For this review, take the finished solid that the model builds, in its own axes (mm). Face numbers are marked on the shaded views. A direction names the side the tool comes from. Round coordinates to 2 decimals unless told otherwise and drop trailing zeros. Loops run counter-clockwise (first coordinate to the right, second up) from the corner with the lowest first, then second, coordinate; pieces in that order, holes last.
```python
from build123d import *
from build123d.topology import SkipClean

# Parameters (mm, degrees)
ESQUISSE1_R             = 17.5
ESQUISSE1_R_2           = 7.5
ESQUISSE1_R_3           = 10
ESQUISSE1_R_4           = 3
BOSS_EXTRU_1_DEPTH      = 11
BOSS_EXTRU_2_DEPTH      = 15.5
BOSS_EXTRU_2_DEPTH_BACK = 4.5
ESQUISSE1_3_R           = 17.5
ESQUISSE1_3_R_2         = 7.5
ESQUISSE1_3_R_3         = 10
ESQUISSE1_3_R_4         = 3


with BuildPart() as part:
    # Esquisse1 → Boss.-Extru.1 (new body)
    # profile 1 of 3: a face of its own
    with BuildSketch(Plane.XY):
        with BuildLine():
            Line((46.99759236, 11.06690166), (2.435529267, 17.329691203))
            ThreePointArc((2.435529267, 17.329691203), (13.207417654, 11.481033007), (17.5, 0))
            ThreePointArc((17.5, 0), (14.881876713, -9.207591731), (7.810886229, -15.660142283))
            Line((7.810886229, -15.660142283), (43.63238408, -12.07959879))
            Line((43.63238408, -12.07959879), (50.273258771, -18.558335793))
            ThreePointArc((50.273258771, -18.558335793), (54.140410924, -6.679083669), (66.578967785, -7.842612783))
            Line((66.578967785, -7.842612783), (46.99759236, 11.06690166))
        make_face()
    # profile 2 of 3: a face of its own
    with BuildSketch(Plane.XY):
        Circle(ESQUISSE1_R)
        Circle(ESQUISSE1_R_2, mode=Mode.SUBTRACT)
    # profile 3 of 3: a face of its own
    with BuildSketch(Plane.XY):
        with Locations((59.63238408, -15.036010787)):
            Circle(ESQUISSE1_R_3)
        with Locations((59.63238408, -15.036010787)):
            Circle(ESQUISSE1_R_4, mode=Mode.SUBTRACT)
    extrude(amount=BOSS_EXTRU_1_DEPTH)

    # Esquisse1_3 → Boss.-Extru.2 (add, two sides: drawn at the far end of the back side and taken through both)
    # profile 1 of 2: a face of its own
    with SkipClean():  # the faces are left unmerged after this step: merging them gives an invalid solid
        with BuildSketch(Plane.XY.offset(-BOSS_EXTRU_2_DEPTH_BACK)):
            Circle(ESQUISSE1_3_R)
            Circle(ESQUISSE1_3_R_2, mode=Mode.SUBTRACT)
        # profile 2 of 2: a face of its own
        with BuildSketch(Plane.XY.offset(-BOSS_EXTRU_2_DEPTH_BACK)):
            with Locations((59.63238408, -15.036010787)):
                Circle(ESQUISSE1_3_R_3)
            with Locations((59.63238408, -15.036010787)):
                Circle(ESQUISSE1_3_R_4, mode=Mode.SUBTRACT)
        extrude(amount=BOSS_EXTRU_2_DEPTH + BOSS_EXTRU_2_DEPTH_BACK)
    add(part.part.scale(1), mode=Mode.REPLACE)  # the faces are merged on a copy


solid = part.part
```
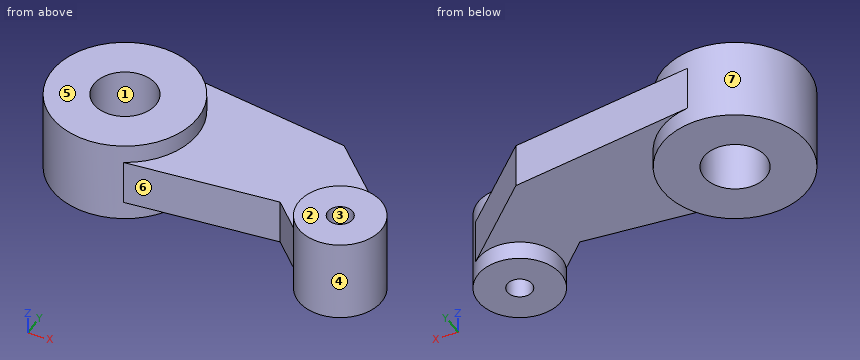
(1) For the marked faces 5, 6 and 7, list the 3-axis set-ups (+Z, -Z, +X, -X, +Y, -Y) from which the entire face can be reached by the end or side of a thin tool; tool diameter is ignored.
(2) Add section A-A (x = 0). Give the boundary of the cut face in (y, z), plus the area to 3 significant figures.
(3) Add section C-C (z = -2.5). Give the boundary of the cut face in (x, y), plus the area to 3 significant figures.
(4) Insertion check: pin 1 Ø1 at (x, z) = (15, -2.5) entering from -Y; pin 2 Ø1.5 at (y, z) = (4, 13.5) entering from +X; pin 3 Ø18 at (x, y) = (28, -7) entering from -Z. Each pin has a flat end and moves straight along its axis. Give the tip position at first contact, or say it passes through.
(5) For L1, parallel to Y at x = 0, z = 3; L2, parallel to X at y = -15.5, z = 12; L3, parallel to X at y = -5, z = -3.25, list the stretches that pass through material, from the lowest coordinate up.
(6) Add section D-D (y = 8.5). Give the boundary of the cut face in (x, z).
(7) The part is to be moulded in two halves that separate along Y. For the marked faces 1, 2, 3 and 4, say which applies: pulls with the +Y half, pulls with the -Y half, needs draft (parallel to the pull), parting line crosses it, or undercut.
(8) Add section B-B (y = 0). Give the boundary of the cut face in (x, z), plus the area to 3 significant figures.
Outcome:
1. face 5: +Z, +X, -X, +Y, -Y
1. face 6: +Z, -Z, -Y
1. face 7: none
2. outline: (-17.5, -4.5) - (-7.5, -4.5) - (-7.5, 15.5) - (-17.5, 15.5) - close; (7.5, -4.5) - (17.5, -4.5) - (17.5, 15.5) - (7.5, 15.5) - close
2. area: 400 mm2
3. outline: circle Ø35 at (0, 0); circle Ø20 at (59.63, -15.04); hole circle Ø15 at (0, 0); hole circle Ø6 at (59.63, -15.04)
3. area: 1,070 mm2
4. pin 1: stops at y = -9.8
4. pin 2: stops at x = 17.2
4. pin 3: stops at z = 0
5. L1: y = -17.5 to -7.5, 7.5 to 17.5
5. L2: x = -8.12 to 8.12, 49.64 to 56.67, 62.6 to 69.62
5. L3: x = -16.77 to -5.59, 5.59 to 16.77
6. outline: (-15.3, -4.5) - (15.3, -4.5) - (15.3, 0) - (49.66, 0) - (49.66, 11) - (15.3, 11) - (15.3, 15.5) - (-15.3, 15.5) - close
7. face 1: undercut
7. face 2: needs draft
7. face 3: undercut
7. face 4: parting line crosses it
8. outline: (-17.5, -4.5) - (-7.5, -4.5) - (-7.5, 15.5) - (-17.5, 15.5) - close; (7.5, -4.5) - (17.5, -4.5) - (17.5, 0) - (58.46, 0) - (58.46, 11) - (17.5, 11) - (17.5, 15.5) - (7.5, 15.5) - close
8. area: 851 mm2
